Design review of the part built by this model. Coordinates are the model's own, in mm. Face numbers are marked on the shaded views. A direction names the side the tool comes from. Round coordinates to 2 decimals unless told otherwise and drop trailing zeros. Write each loop counter-clockwise with the first axis right and the second up, starting at its lowest first coordinate (ties: lowest second). Pieces come first, ordered by that corner, then holes. Notation, with made-up numbers: M -33,83.5 L 12,83.5 A14 cw 12,93.5 Z; hole C -31.75,64 d4. An arc over 180 degrees is marked long. Use CSV: the item, a comma, the result in double quotes.
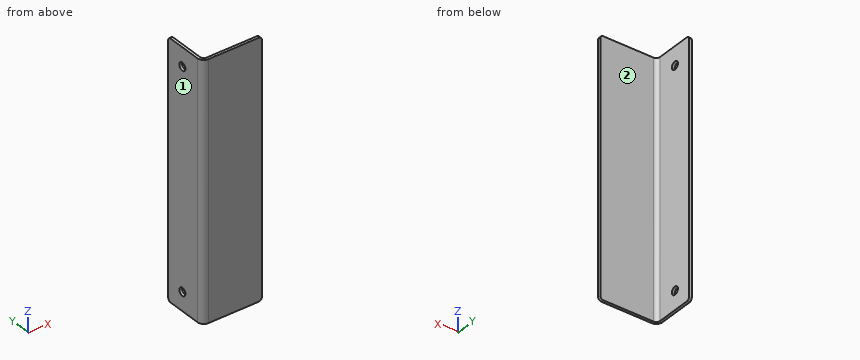
from build123d import *

# Parameters (mm, degrees)
SKETCH1_W                    = 38.1
SKETCH1_H                    = 215.9
BASE_FLANGE1_DEPTH           = 2.304796
EDGE_FLANGE1_STRIP_W         = 15.219184
EDGE_FLANGE1_STRIP_H         = 2.304796
EDGE_FLANGE1_STRIP_CUT_DEPTH = 215.9
EDGE_FLANGE1_DEPTH           = 215.9
F_1_4_CLEARANCE_HOLE1_D      = 6.7564
FILLET1_R                    = 2.54


# Sheet-metal steps are written as plain solids
with BuildPart() as part:
    # Sketch1 → Base-Flange1 (new body)
    with BuildSketch(Plane(origin=(0, 0, 0), x_dir=(0, -1, 0), z_dir=(1, 0, 0))):
        with Locations((-19.05, -107.95)):
            Rectangle(SKETCH1_W, SKETCH1_H)
    extrude(amount=-BASE_FLANGE1_DEPTH)

    # Edge-Flange1 strip (across the edge) → Edge-Flange1 strip cut (cut)
    with BuildSketch(Plane.YX.offset(-215.9)):
        with Locations((-2.304796, -1.152398)):
            Rectangle(EDGE_FLANGE1_STRIP_W, EDGE_FLANGE1_STRIP_H)
    extrude(amount=EDGE_FLANGE1_STRIP_CUT_DEPTH, mode=Mode.SUBTRACT)

    # Edge-Flange1 section (across the edge) → Edge-Flange1 (add)
    with BuildSketch(Plane.YX.offset(-215.9)):
        with BuildLine():
            Line((0, 3), (0, 48.495204))
            Line((0, 48.495204), (2.304796, 48.495204))
            Line((2.304796, 48.495204), (2.304796, 3))
            ThreePointArc((2.304796, 3), (3.183475656, 0.878679656), (5.304796, 0))
            Line((5.304796, 0), (5.304796, -2.304796))
            ThreePointArc((5.304796, -2.304796), (1.553738776, -0.751057224), (0, 3))
        make_face()
    extrude(amount=EDGE_FLANGE1_DEPTH)

    # 1/4 Clearance Hole1 (through all)
    with Locations(Plane.ZY.offset(2.304796)):
        with Locations((15.875, 22.225), (200.025, 22.225)):
            Hole(F_1_4_CLEARANCE_HOLE1_D / 2)

    # Fillet1
    fillet1_edges = [part.edges().sort_by_distance(p)[0] for p in [
        (48.495204, 1.152398, 215.9),
        (48.495204, 1.152398, 0),
        (-1.152398, 38.1, 215.9),
        (-1.152398, 38.1, 0),
    ]]
    fillet(fillet1_edges, radius=FILLET1_R)


solid = part.part
1) Add section B-B on x = 32. Write out the cut boundary in (y, z).
Answers:
outline,"M 0,0 L 2.3,0 L 2.3,215.9 L 0,215.9 Z"
2) For pin 1 Ø5 at (y, z) = (31, 55) entering from +X; pin 2 Ø2 at (x, z) = (32, 121) entering from +Y, all flat-tipped, find the tip position at first contact; note any pin that passes through.
Answers:
pin 1,"x = 0"
pin 2,"y = 2.3"
3) Machinability: for the marked faces 1 and 2, which of the approach directions +Z, -Z, +X, -X, +Y, -Y give a long, thin tool a straight path to every point of the face, cutting with its end or side? Answer none if there is none.
Answers:
face 1,"+Z, -Z, -X, +Y, -Y"
face 2,"+Z, -Z, +X, +Y"
4) Wall thickness on line 1 along X through (y, z) = (14.5, 53); line 2 along Y through (x, z) = (44.5, 156.5): over which ranges is each line inside the solid? List them lowest first. Write a range as [from, to].
Answers:
line 1,"[-2.3, 0]"
line 2,"[0, 2.3]"
5) Add section A-A on z = 45. Write out the cut boundary in (x, y), then the cut area to 3 significant figures.
Answers:
outline,"M -2.3,5.3 A5.3 ccw 3,0 L 48.5,0 L 48.5,2.3 L 3,2.3 A3 cw 0,5.3 L 0,38.1 L -2.3,38.1 Z"
area,"195 mm²"
6) Add section C-C on y = 27.5. Write out the cut boundary in (x, z).
Answers:
outline,"M -2.3,0 L 0,0 L 0,215.9 L -2.3,215.9 Z"
